Work out the finished part from the listing and answer in its coordinate system (mm). A direction names the side the tool comes from. Give positions to 0.01 mm unless a question says otherwise; leave off trailing zeros. Write each loop counter-clockwise with the first axis right and the second up, starting at its lowest first coordinate (ties: lowest second). Pieces come first, ordered by that corner, then holes. Notation, with made-up numbers: (48, 50) - (57, 50) arc R8 cw to (57, 58) - close; hole circle Ø10 at (52.25, 69). An arc over 180 degrees is marked (long way). Write item = value, one per line.
from build123d import *

# Parameters (mm, degrees)
F0_W     = 40
F0_H     = 25
F1_DEPTH = 5
F2_W     = 8
F2_H     = 3
F3_DEPTH = 8
F4_R     = 3
F6_DEPTH = 25


with BuildPart() as f1:
    # F0 (on Top) → F1 (new body)
    with BuildSketch(Plane.XY):
        Rectangle(F0_W, F0_H)
    extrude(amount=F1_DEPTH)

    # F2 (on face) → F3 (join)
    with BuildSketch(Plane.XY.offset(5)):
        with Locations((12.6486493205, 6)):
            Rectangle(F2_W, F2_H)
        with Locations((12.6486493205, 0)):
            Rectangle(F2_W, F2_H)
        with Locations((12.6486493205, -6)):
            Rectangle(F2_W, F2_H)
    extrude(amount=F3_DEPTH)

    # F4
    f4_edges = [f1.edges().sort_by_distance(p)[0] for p in [
        (8.648649, -6, 13),
        (16.648649, -6, 13),
        (8.648649, 0, 13),
        (16.648649, 0, 13),
        (8.648649, 6, 13),
        (16.648649, 6, 13),
    ]]
    fillet(f4_edges, radius=F4_R)

    # F5 (on face) → F6 (cut)
    with BuildSketch(Plane.XZ.offset(7.5)):
        with BuildLine():
            ThreePointArc((14.1486493205, 10), (13.7093094923, 11.0606601718), (12.6486493205, 11.5))
            ThreePointArc((12.6486493205, 11.5), (11.5879891487, 8.9393398282), (14.1486493205, 10))
        make_face()
    extrude(amount=-F6_DEPTH, mode=Mode.SUBTRACT)


solid = f1.part
1. A tool of negligible diameter and unlimited length cuts with its end or side. For faces 1 (the flat face through (13, 4.5, 8)), 2 (the flat face through (16.649, -6, 7)), 3 (the flat face through (8.649, 6, 7)), 4 (the flat face through (13, -7.5, 8)), from which of +Z, -Z, +X, -X, +Y, -Y can it reach the whole face along a straight path? Write none if from no direction.
Solution:
face_1 = +Z, +X, -X
face_2 = +Z, +X, +Y, -Y
face_3 = +Z, -X, +Y, -Y
face_4 = +Z, +X, -X, -Y
2. Given pin 1 (0.9 mm diameter, centred on y = -5.5, z = 7.5, fed in from +X); pin 2 (2.5 mm diameter, centred on y = -5.5, z = 8, fed in from -X); pin 3 (4 mm diameter, centred on x = 11.5, z = 8, fed in from +Y), each flat-ended and moving along its own axis, determine where each tip first touches the part or whether it passes through.
Solution:
pin_1 = 16.65
pin_2 = 8.65
pin_3 = 7.5
3. Find section B-B, the plane x = -5. Give the vertices of the cut face in (y, z), then the cut area to 3 significant figures.
Solution:
outline = (-12.5, 0) - (12.5, 0) - (12.5, 5) - (-12.5, 5) - close
area = 125 mm^2
4. Find section C-C, the plane y = 2.25. Give the vertices of the cut face in (x, z).
Solution:
outline = (-20, 0) - (20, 0) - (20, 5) - (-20, 5) - close
5. Straight lines are drawn through the part: line 1 (Y direction, x = 16.5, z = 10); line 2 (X direction, y = 5.75, z = 10); line 3 (Z direction, x = 9.5, y = 8). For each, find the intervals that lie inside material, in ascending order.
Solution:
line_1 = -7.5 to -4.5, -1.5 to 1.5, 4.5 to 7.5
line_2 = 8.65 to 11.15, 14.15 to 16.65
line_3 = 0 to 5
6. For a pull along Y with two mould halves and no side action, classify faces 5 (the flat face through (0, 0, 0)), 6 (the flat face through (0, -12.5, 2)), 7 (the flat face through (13, -4.5, 8)) as pulls with the +Y half, pulls with the -Y half, needs draft (parallel to the pull), parting line crosses it, or undercut.
Solution:
face_5 = needs draft
face_6 = pulls with the -Y half
face_7 = undercut
7. Find section A-A, the plane z = 8. Give the vertices of the cut face in (x, y), then the cut area to 3 significant figures.
Solution:
outline = (8.65, -7.5) - (16.65, -7.5) - (16.65, -4.5) - (8.65, -4.5) - close; (8.65, -1.5) - (16.65, -1.5) - (16.65, 1.5) - (8.65, 1.5) - close; (8.65, 4.5) - (16.65, 4.5) - (16.65, 7.5) - (8.65, 7.5) - close
area = 72.0 mm^2
